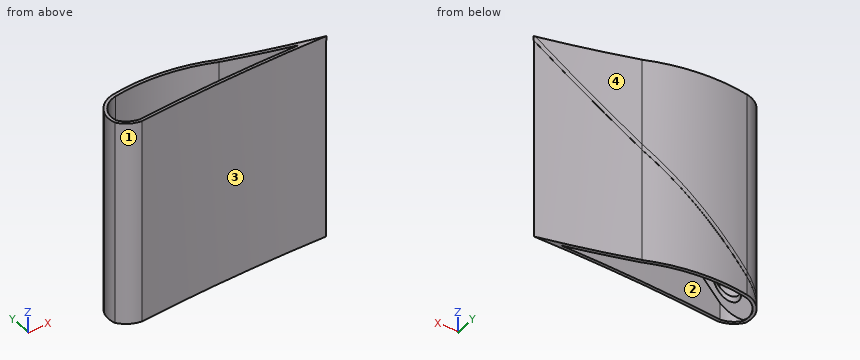
```python
from build123d import *

# Parameters (mm, degrees)
F3_DEPTH = 100
F4_DEPTH = 25
F2_W     = 130.920828
F2_H     = 57.169587
F5_DEPTH = 100
F6_R     = 5.5
F6_R_2   = 4
F6_R_3   = 2.5
F7_DEPTH = 100


with BuildPart() as f3:
    # F0 (on Top) → F3 (new body)
    with BuildSketch(Plane.XY):
        with BuildLine():
            ThreePointArc((-50.955394, 8.962345), (-50.814737, 7.217467), (-50.396399, 5.517649))
            ThreePointArc((-50.396399, 5.517649), (-46.499614, 1.806953), (-41.431171, 0))
            ThreePointArc((-41.431171, 0), (3.806717, 1.130986), (49.044606, 0))
            ThreePointArc((49.044606, 0), (27.138267, 6.303353), (5.490228, 13.443548))
            ThreePointArc((5.490228, 13.443548), (-17.086444, 20.012497), (-40.598205, 20.245597))
            ThreePointArc((-40.598205, 20.245597), (-46.578725, 17.678098), (-50.396399, 12.407041))
            ThreePointArc((-50.396399, 12.407041), (-50.814737, 10.707224), (-50.955394, 8.962345))
        make_face()
        with BuildLine():
            ThreePointArc((-40.401325, 18.758555), (-17.271527, 18.523557), (4.934787, 12.048809))
            ThreePointArc((4.934787, 12.048809), (20.441613, 6.838342), (36.085862, 2.056282))
            ThreePointArc((36.085862, 2.056282), (-2.645042, 2.608034), (-41.364174, 1.505217))
            ThreePointArc((-41.364174, 1.505217), (-45.679897, 3.063858), (-49.037404, 6.191472))
            ThreePointArc((-49.037404, 6.191472), (-49.45495, 9.05371), (-48.981805, 11.907284))
            ThreePointArc((-48.981805, 11.907284), (-45.633862, 16.513045), (-40.401325, 18.758555))
        make_face(mode=Mode.SUBTRACT)
    extrude(amount=F3_DEPTH)

    # F1 (on Front) → F4 (join)
    with BuildSketch(Plane.XZ):
        Polygon((-50.949167, 1.414214), (-50.949167, 0), (-49.534954, 0), (49.050833, 98.585786), (49.050833, 100), (47.636619, 100), align=None)
    extrude(amount=-F4_DEPTH)

    # F2 (on Top) → F5 (cut)
    with BuildSketch(Plane.XY):
        with Locations((0.042133, 7.232606)):
            Rectangle(F2_W, F2_H)
        with BuildLine():
            ThreePointArc((-41.397933, 0.104339), (-46.4615, 1.912404), (-50.354612, 5.62084))
            ThreePointArc((-50.354612, 5.62084), (-50.907918, 9.032238), (-50.354612, 12.443636))
            ThreePointArc((-50.354612, 12.443636), (-46.537025, 17.713711), (-40.557266, 20.28084))
            ThreePointArc((-40.557266, 20.28084), (-17.07095, 20.047617), (5.481051, 13.484941))
            ThreePointArc((5.481051, 13.484941), (26.810456, 6.442957), (48.391087, 0.213235))
            ThreePointArc((48.391087, 0.213235), (3.495226, 1.272535), (-41.397933, 0.104339))
        make_face(mode=Mode.SUBTRACT)
    extrude(amount=F5_DEPTH, mode=Mode.SUBTRACT)

    # F6 (on Top) → F7 (cut)
    with BuildSketch(Plane.XY):
        with Locations((-38.668361, 9.792585)):
            Circle(F6_R)
        with Locations((-22.44026, 9.580453)):
            Circle(F6_R)
        with Locations((-6.742489, 9.156189)):
            Circle(F6_R_2)
        with Locations((5.561169, 6.928802)):
            Circle(F6_R_3)
    extrude(amount=F7_DEPTH, mode=Mode.SUBTRACT)


solid = f3.part
```
Read the model definition and answer for the solid it produces. Units are mm, in the model's axes. Face numbers are marked on the shaded views. Coordinates: 2 decimals unless noted, no trailing zeros.
(1) The mould has two halves that part along X. Classify the marked faces 1, 2, 3 and 4: released by +X, released by -X, zero draft, split by the parting line, or undercut.
Solution:
face 1: released by -X
face 2: undercut
face 3: undercut
face 4: released by +X
(2) The part is cut by section A-A (z = 83.5). Count the separate pieces of the cut face and the enclosed holes in it, and give its area (3 significant figures).
Solution:
separate pieces: 1
enclosed holes: 2
area: 286 mm2
(3) Consider line 1 along Y through (x, z) = (-6.5, 92.5); line 2 along Y through (x, z) = (10.5, 7); line 3 along Z through (x, y) = (9, 4). Determine where each line is inside the solid, lowest interval first.
Solution:
line 1: y = 1.21 to 2.57, 16.21 to 17.76
line 2: y = 1.25 to 2.61, 10.12 to 11.71
line 3: z = 58.53 to 61.36
(4) Flat-ended cylindrical pins translate along their axes: pin 1 Ø12 at (x, y) = (-22.5, 17.5) entering from -Z; pin 2 Ø4 at (x, z) = (-8.5, 78) entering from -Y; pin 3 Ø6.5 at (x, y) = (-22.44, 9.58) entering from +Z; pin 4 Ø12 at (x, z) = (12, 83) entering from -Y. Find the tip coordinate at first contact, or state that the pin passes through.
Solution:
pin 1: stops at z = 0
pin 2: stops at y = 1.15
pin 3: passes through
pin 4: stops at y = 1.17
